Verification items for this drawing (mm, ordinates from the low corner). Round coordinates to 2 decimals unless told otherwise and drop trailing zeros. Order: outer loops, then holes, each group sorted by start corner. A loop starts at its lowest first (then second) coordinate and runs counter-clockwise, first axis right, second up. Notation, with made-up numbers: (-23, -19) -> (-11, -19) arc R24 ccw to (-11, 3) -> close; hole circle Ø3 at (51.5, 1). An arc over 180 degrees is marked (long way). Put each result on its own line as item: value.
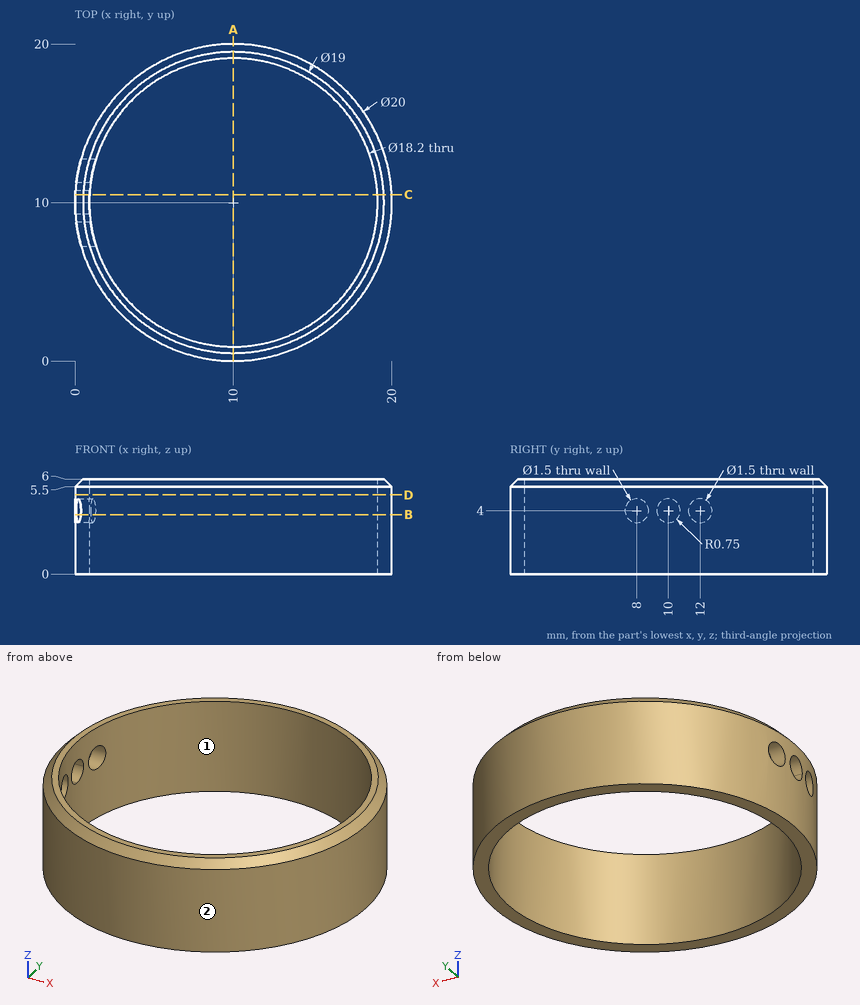
Item 1: Section check B-B on z = 3.75. Record the boundary of the cut face in (x, y).
Check sheet entries:
outline: (0.03, 9.29) arc R10 ccw to (0.08, 8.71) -> (0.99, 8.71) arc R9.1 cw to (0.93, 9.29) -> close; (0.03, 10.71) -> (0.93, 10.71) arc R9.1 cw to (0.99, 11.29) -> (0.08, 11.29) arc R10 ccw to start; (0.37, 7.29) arc R10 ccw (long way) to (0.37, 12.71) -> (1.31, 12.71) arc R9.1 cw (long way) to (1.31, 7.29) -> close
Item 2: Section check D-D on z = 5. Record the boundary of the cut face in (x, y), then the cut area to 3 significant figures.
Check sheet entries:
outline: circle Ø20 at (10, 10); hole circle Ø18.2 at (10, 10)
area: 54.0 mm^2
Item 3: Section check C-C on y = 10.5. State how many separate pieces and enclosed holes the cut face has, then the cut area to 3 significant figures.
Check sheet entries:
separate pieces: 3
enclosed holes: 0
area: 9.56 mm^2
Item 4: Material ranges on L1, parallel to Y at x = 10, z = 2; L2, parallel to X at y = 9.5, z = 2.25; L3, parallel to Y at x = 1.75, z = 4.5, recorded low to high. Write a range as [from, to].
Check sheet entries:
L1: y = [0, 0.9], [19.1, 20]
L2: x = [0.01, 0.91], [19.09, 19.99]
L3: y = [4.35, 6.16], [13.84, 15.65]
Item 5: Section check A-A on x = 10. Record the boundary of the cut face in (y, z).
Check sheet entries:
outline: (0, 0) -> (0.9, 0) -> (0.9, 6) -> (0.5, 6) -> (0, 5.5) -> close; (19.1, 0) -> (20, 0) -> (20, 5.5) -> (19.5, 6) -> (19.1, 6) -> close
Item 6: Release check for a two-part mould opening along Y. For the marked faces 1 and 2 record: +Y half, -Y half, draft (parallel to the pull), parting line (faces both ways), or undercut.
Check sheet entries:
face 1: undercut
face 2: parting line
Item 7: Gauge pin test, flat ends, axial feed: pin 1 Ø1.2 at (y, z) = (12, 4) entering from +X; pin 2 Ø1.5 at (x, z) = (2.5, 5) entering from -Y. Record the tip position at first contact, or that the pin passes through.
Check sheet entries:
pin 1: stops at x = 19.9
pin 2: stops at y = 2.62
